Input: part model. Units: mm. Frame: model coordinates. Face numbers are marked on the shaded views. A direction names the side the tool comes from. Coordinates: 2 decimals unless noted, no trailing zeros. Write each loop counter-clockwise with the first axis right and the second up, starting at its lowest first coordinate (ties: lowest second). Pieces come first, ordered by that corner, then holes. Notation, with made-up numbers: (-13, -37) - (31, -37) arc R21 cw to (31, -9) - close; hole circle Ø4 at (31.5, 28.5). An arc over 180 degrees is marked (long way). Put each result on its own line as item: value. Start each with the question number.
1. Pin query (flat end, axial travel): pin 1 (1.6 mm diameter, centred on y = 0.5, z = -26, fed in from +X); pin 2 (12 mm diameter, centred on x = -57, z = -56.5, fed in from -Y). Return the tip coordinate at first contact, or that it passes through.
2. Cut plane B-B, the plane x = 9.5. Return loops of the section in (y, z).
3. Access query for the marked faces 1 and 2. Directions: +Z, -Z, +X, -X, +Y, -Y. A direction counts if a zero-diameter tool reaches every point of the face in a straight line with its end or side. Return the directions, or none.
4. Cut plane D-D, the plane x = -38.5. Return loops of the section in (y, z), and give its area (3 significant figures).
5. Cut plane A-A, the plane y = 1.35. Return loops of the section in (x, z).
6. Cut plane C-C, the plane x = -63.25. Return loops of the section in (y, z) (3 decimals), and give its area (3 significant figures).
7. Pull-direction query (Z, two-part tool) for the marked faces 3 and 4; classes: released by +Z, released by -Z, zero draft, split by the parting line, or undercut.
8. Line query: line 1 (Z direction, x = -53, y = 1.4); line 2 (X direction, y = 0.4, z = -61); line 3 (Z direction, x = -45.75, y = 2.8) (1 decimal). Output: solid intervals per line, ascending.
from build123d import *

# Parameters (mm, degrees)
ESQUISSE1_W              = 148
ESQUISSE1_H              = 148
BOSS_EXTRU_1_DEPTH       = 4
ESQUISSE4_R              = 1.8
ENL_V_MAT_EXTRU_2_DEPTH  = 4
ESQUISSE5_W              = 35.5
ESQUISSE5_H              = 23.5
ENL_V_MAT_EXTRU_3_DEPTH  = 2
ESQUISSE8_R              = 1.8
ENL_V_MAT_EXTRU_6_DEPTH  = 4
ESQUISSE9_W              = 35.5
ESQUISSE9_H              = 23.5
ENL_V_MAT_EXTRU_7_DEPTH  = 2
ESQUISSE10_R             = 1.8
ENL_V_MAT_EXTRU_8_DEPTH  = 4
ESQUISSE11_W             = 35.5
ESQUISSE11_H             = 23.5
ESQUISSE11_H_2           = 23.512269398
ENL_V_MAT_EXTRU_9_DEPTH  = 2
ESQUISSE12_W             = 23.640980831
ESQUISSE12_H             = 10
ESQUISSE12_W_2           = 17.131931469
ENL_V_MAT_EXTRU_12_DEPTH = 2


with BuildPart() as part:
    # Esquisse1 → Boss.-Extru.1 (new body)
    with BuildSketch(Plane(origin=(0, 0, 0), x_dir=(1, 0, 0), z_dir=(0, 1, 0))):
        Rectangle(ESQUISSE1_W, ESQUISSE1_H)
    extrude(amount=BOSS_EXTRU_1_DEPTH)

    # Esquisse4 → Enlèv. mat.-Extru.2 (cut)
    with BuildSketch(Plane(origin=(0, 0, 0), x_dir=(1, 0, 0), z_dir=(0, 1, 0))):
        with Locations((-63.25, -60.525)):
            Circle(ESQUISSE4_R)
        with Locations((-45.75, -60.525)):
            Circle(ESQUISSE4_R)
    extrude(amount=ENL_V_MAT_EXTRU_2_DEPTH, mode=Mode.SUBTRACT)

    # Esquisse5 → Enlèv. mat.-Extru.3 (cut)
    with BuildSketch(Plane(origin=(0, 0, 0), x_dir=(1, 0, 0), z_dir=(0, 1, 0))):
        with Locations((-54.25, -60.25)):
            Rectangle(ESQUISSE5_W, ESQUISSE5_H)
    extrude(amount=ENL_V_MAT_EXTRU_3_DEPTH, mode=Mode.SUBTRACT)

    # Esquisse8 → Enlèv. mat.-Extru.6 (cut)
    with BuildSketch(Plane(origin=(0, 0, 0), x_dir=(1, 0, 0), z_dir=(0, 1, 0))):
        with Locations((-2.725, -60.525)):
            Circle(ESQUISSE8_R)
        with Locations((14.825, -60.525)):
            Circle(ESQUISSE8_R)
    extrude(amount=ENL_V_MAT_EXTRU_6_DEPTH, mode=Mode.SUBTRACT)

    # Esquisse9 → Enlèv. mat.-Extru.7 (cut)
    with BuildSketch(Plane(origin=(0, 0, 0), x_dir=(1, 0, 0), z_dir=(0, 1, 0))):
        with Locations((6.25, -60.25)):
            Rectangle(ESQUISSE9_W, ESQUISSE9_H)
    extrude(amount=ENL_V_MAT_EXTRU_7_DEPTH, mode=Mode.SUBTRACT)

    # Esquisse10 → Enlèv. mat.-Extru.8 (cut)
    with BuildSketch(Plane(origin=(0, 0, 0), x_dir=(1, 0, 0), z_dir=(0, 1, 0))):
        with Locations((-2.725, 60.525)):
            Circle(ESQUISSE10_R)
        with Locations((14.825, 60.525)):
            Circle(ESQUISSE10_R)
        with Locations((-63.125, 60.525)):
            Circle(ESQUISSE10_R)
        with Locations((-45.375, 60.525)):
            Circle(ESQUISSE10_R)
    extrude(amount=ENL_V_MAT_EXTRU_8_DEPTH, mode=Mode.SUBTRACT)

    # Esquisse11 → Enlèv. mat.-Extru.9 (cut)
    with BuildSketch(Plane(origin=(0, 0, 0), x_dir=(1, 0, 0), z_dir=(0, 1, 0))):
        with Locations((-54.25, 60.25)):
            Rectangle(ESQUISSE11_W, ESQUISSE11_H)
        with Locations((6.25, 60.243865301)):
            Rectangle(ESQUISSE11_W, ESQUISSE11_H_2)
    extrude(amount=ENL_V_MAT_EXTRU_9_DEPTH, mode=Mode.SUBTRACT)

    # Esquisse12 → Enlèv. mat.-Extru.12 (cut)
    with BuildSketch(Plane(origin=(0, 0, 0), x_dir=(1, 0, 0), z_dir=(0, 1, 0))):
        with Locations((68.740682109, -25.384218458)):
            Rectangle(ESQUISSE12_W, ESQUISSE12_H)
        with Locations((65.486157429, 24.615781542)):
            Rectangle(ESQUISSE12_W_2, ESQUISSE12_H)
    extrude(amount=ENL_V_MAT_EXTRU_12_DEPTH, mode=Mode.SUBTRACT)


solid = part.part
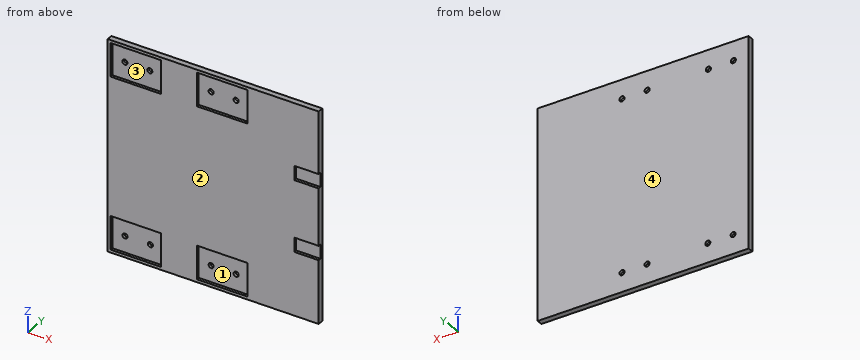
Report:
1. pin 1: stops at x = 56.92
1. pin 2: stops at y = 2
2. outline: (0, -74) - (4, -74) - (4, 74) - (0, 74) - (0, 72) - (2, 72) - (2, 48.5) - (0, 48.5) - (0, -48.49) - (2, -48.49) - (2, -72) - (0, -72) - close
3. face 1: -Y
3. face 2: +Z, -Z, +X, -X, -Y
4. outline: (0, -74) - (4, -74) - (4, 74) - (0, 74) - (0, 72) - (2, 72) - (2, 48.5) - (0, 48.5) - (0, -48.5) - (2, -48.5) - (2, -72) - (0, -72) - close
4. area: 498 mm^2
5. outline: (-74, -74) - (74, -74) - (74, -29.62) - (56.92, -29.62) - (56.92, -19.62) - (74, -19.62) - (74, 20.38) - (56.92, 20.38) - (56.92, 30.38) - (74, 30.38) - (74, 74) - (-74, 74) - close; hole (-72, -72) - (-36.5, -72) - (-36.5, -48.5) - (-72, -48.5) - close; hole (-72, 48.5) - (-36.5, 48.5) - (-36.5, 72) - (-72, 72) - close; hole (-11.5, -72) - (24, -72) - (24, -48.49) - (-11.5, -48.49) - close; hole (-11.5, 48.5) - (24, 48.5) - (24, 72) - (-11.5, 72) - close
6. outline: (0, -74) - (4, -74) - (4, -62.321) - (2, -62.321) - (2, -72) - (0, -72) - close; (0, -48.5) - (2, -48.5) - (2, -58.729) - (4, -58.729) - (4, 58.725) - (2, 58.725) - (2, 48.5) - (0, 48.5) - close; (0, 72) - (2, 72) - (2, 62.325) - (4, 62.325) - (4, 74) - (0, 74) - close
6. area: 484 mm^2
7. face 3: undercut
7. face 4: zero draft
8. line 1: z = -74 to -72, -48.5 to 48.5, 72 to 74
8. line 2: x = -74 to -72, -36.5 to -11.5, 24 to 74
8. line 3: z = -74 to -62.3, -58.8 to 58.7, 62.3 to 74
